Here's the drawing with two shaded views (mm, measured from the low corner). I have some questions. A direction names the side the tool comes from. Round coordinates to 2 decimals unless told otherwise and drop trailing zeros. Write each loop counter-clockwise with the first axis right and the second up, starting at its lowest first coordinate (ties: lowest second). Pieces come first, ordered by that corner, then holes. Notation, with made-up numbers: (-9, 34) -> (43, 34) arc R29 ccw to (43, 64) -> close; hole circle Ø5 at (-30, 33). An arc over 180 degrees is marked (long way). Use CSV: the item, a comma, the result in double quotes.
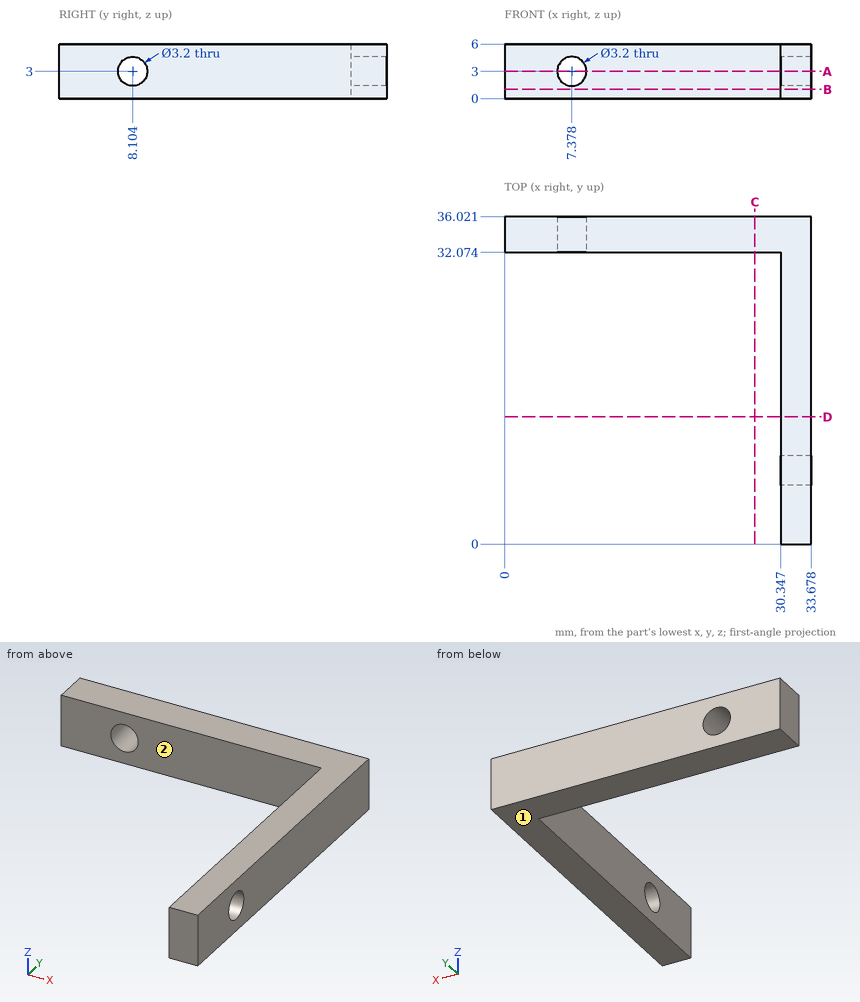
Q1. Please list where these lines run through material, in increasing order: probe 1 along Y at (x, z) = (31.2, 3) (1 decimal); probe 2 along Y at (x, z) = (11.5, 1.1); probe 3 along X at (y, z) = (6, 4.55).
Resolved:
probe 1,"y = 0 to 6.5, 9.7 to 36"
probe 2,"y = 32.07 to 36.02"
probe 3,"x = 30.35 to 33.68"
Q2. Suppose I cut it at A-A (z = 3). Write out the boundary of the cut face in (x, y) (1 decimal).
Resolved:
outline,"(0, 32.1) -> (5.8, 32.1) -> (5.8, 36) -> (0, 36) -> close; (9, 32.1) -> (30.3, 32.1) -> (30.3, 9.7) -> (33.7, 9.7) -> (33.7, 36) -> (9, 36) -> close; (30.3, 0) -> (33.7, 0) -> (33.7, 6.5) -> (30.3, 6.5) -> close"
Q3. Suppose I cut it at B-B (z = 1). Write out the boundary of the cut face in (x, y).
Resolved:
outline,"(0, 32.07) -> (30.35, 32.07) -> (30.35, 0) -> (33.68, 0) -> (33.68, 36.02) -> (0, 36.02) -> close"
Q4. Suppose I cut it at C-C (x = 27.5). Write out the boundary of the cut face in (y, z), and give its area (3 significant figures).
Resolved:
outline,"(32.07, 0) -> (36.02, 0) -> (36.02, 6) -> (32.07, 6) -> close"
area,"23.7 mm^2"
Q5. Suppose I cut it at D-D (y = 14). Write out the boundary of the cut face in (x, z).
Resolved:
outline,"(30.35, 0) -> (33.68, 0) -> (33.68, 6) -> (30.35, 6) -> close"
Q6. Will these pins go through, and if not, where does the flat tip stop? P1, Ø1, axis at x = 24.5, z = 2.5, coming from the -Y side; P2, Ø3, axis at y = 20.5, z = 5, coming from the -X side.
Resolved:
P1,"stops at y = 32.07"
P2,"stops at x = 30.35"
Q7. On a 3-axis mill with a long thin cutter (end or side, diameter ignored), from which of +Z, -Z, +X, -X, +Y, -Y can I reach the whole of each face in a straight line? I mean the marked faces 1 and 2. Say none if no direction works.
Resolved:
face 1,"-Z, +X, -X, +Y, -Y"
face 2,"+Z, -Z, -X, -Y"
